Autodesk Inventor part; units mm, degrees
ref_plane "YZ Plane" through (0, 0, 0) normal (1, 0, 0) x (0, 1, 0)
ref_plane "XZ Plane" through (0, 0, 0) normal (0, 1, 0) x (-1, 0, 0)
ref_plane "XY Plane" through (0, 0, 0) normal (0, 0, 1) x (1, 0, 0)
sketch "Sketch2" plane through (0, 0, 0) normal (0, 1, 0) x (-1, 0, 0)
  line L0 (0, 0) -> (-30, 0)
  line L1 (-30, 0) -> (-30, -144)
  line L2 (-30, -144) -> (0, -144)
  line L3 (0, -144) -> (0, 0)
  line L4 (0, 0) -> (7, 0)
  line L5 (7, 0) -> (7, -5)
  arc A0 (7, -5) -> (0, -20.1987) centre (20, -20.1987) ccw
  line L6 (0, -144) -> (7, -144)
  line L7 (7, -144) -> (7, -139)
  arc A1 (0, -123.8013) -> (7, -139) centre (20, -123.8013) ccw
  line L8 (-30, 0) -> (-35, 0)
  line L9 (-35, 0) -> (-35, -52)
  line L10 (-35, -52) -> (-30, -52)
  line L11 (-30, -52) -> (-30, 0)
  line L12 (-30, -144) -> (-35, -144)
  line L13 (-35, -144) -> (-35, -92)
  line L14 (-35, -92) -> (-30, -92)
  line L15 (-30, -92) -> (-30, -144)
  line L16 (5, -32) -> (0, -32)
  line L17 (0, -52) -> (5, -52)
  line L18 (5, -52) -> (5, -32)
  line L19 (5, -92) -> (0, -92)
  line L20 (0, -112) -> (5, -112)
  line L21 (5, -112) -> (5, -92)
  dimension "d0" = 144
  dimension "d1" = 30
  dimension "d2" = 5
  dimension "d3" = 7
  dimension "d4" = 20
  dimension "d5" = 7
  dimension "d6" = 5
  dimension "d9" = 20
  dimension "d10" = 5
  dimension "d11" = 5
  dimension "d12" = 40
  dimension "d13" = 40
  dimension "d14" = 5
  dimension "d15" = 5
  dimension "d16" = 20
  dimension "d17" = 20
extrude "Cuerpo" add sketch "Sketch2" along normal blind 3
equation "\"d0\" = deslizador_largo"
equation "\"d1\" = deslizador_ancho"
equation "\"d2\" = deslizador_interruptor_largo"
equation "\"d3\" = deslizador_interruptor_ancho"
equation "\"d4\" = deslizador_interruptor_angulo"
equation "\"d5\" = d3"
equation "\"d6\" = d2"
equation "\"d9\" = d4"
equation "\"d10\" = deslizador_saliente"
equation "\"d11\" = d10"
equation "\"d12\" = movimiento_deslizador + deslizador_tope_largo"
equation "\"d13\" = d12"
equation "\"d14\" = d10"
equation "\"d15\" = d10"
equation "\"d16\" = deslizador_saliente_largo"
equation "\"d17\" = d16"
equation "\"d18\" = deslizador_alto"
equation "\"margen\" = 0.3"
equation "\"base_alto\" = 3"
equation "\"muros_grosor\" = 3"
equation "\"rail_alto\" = 1.5"
equation "\"rail_grosor\" = 5"
equation "\"hoja_stop_posicion\" = 5"
equation "\"hoja_stop_saliente\" = 5"
equation "\"hoja_stop_largo\" = 5"
equation "\"hoja_alto\" = 3"
equation "\"hoja_stop_biselado\" = 2"
equation "\"hoja_filo_biselado\" = 0.5"
equation "\"hoja_cola_biselado\" = 1"
equation "\"deslizador_soporte_alto\" = 4"
equation "\"deslizador_tope_alto\" = 5"
equation "\"deslizador_soporte_ancho\" = 5"
equation "\"deslizador_tope_largo\" = 10"
equation "\"deslizador_alto\" = 3"
equation "\"tirador_agarre_largo\" = 3"
equation "\"movimiento_deslizador\" = 30"
equation "\"deslizador_largo\" = 144"
equation "\"deslizador_ancho\" = 30"
equation "\"deslizador_saliente\" = 5"
equation "\"deslizador_interruptor_angulo\" = 20"
equation "\"deslizador_interruptor_largo\" = 5"
equation "\"deslizador_interruptor_ancho\" = 7"
equation "\"deslizador_saliente_largo\" = 20"
equation "\"traba_top_alto\" = 3"
equation "\"traba_top_largo\" = 5"
equation "\"traba_alto\" = 4"
equation "\"traba_ancho\" = 3"
equation "\"traba_largo\" = 39"
equation "\"traba_diametro\" = 5"
equation "\"traba_diametro_perforacion\" = 2"
equation "\"base_separacion_agujeros\" = 4"
equation "\"base_agujeros_separacion\" = 3.5"
equation "\"base_agujeros_diametro\" = 2"
properties part number "Deslizador"
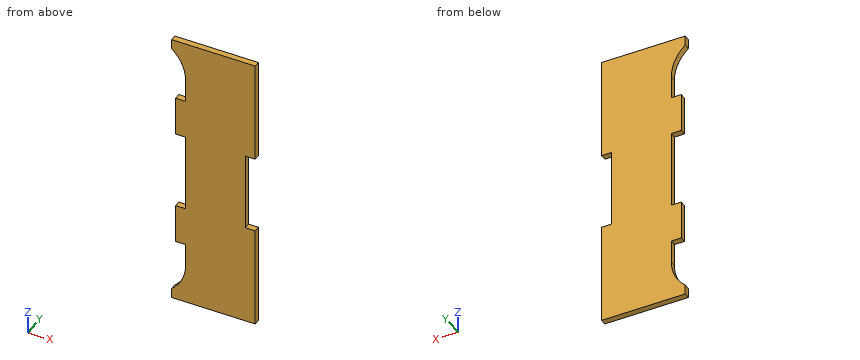
Geometry check sheet. Reference: the model listing, model coordinates, mm. Give positions to 0.01 mm unless a question says otherwise; leave off trailing zeros. Order: outer loops, then holes, each group sorted by start corner. A loop starts at its lowest first (then second) coordinate and runs counter-clockwise, first axis right, second up. Notation, with made-up numbers: (75, 43) - (115, 43) arc R22 ccw to (115, 49) - close; hole circle Ø5 at (-14, -38.5). An arc over 180 degrees is marked (long way). Answer as a JSON object with one key per item and string values.
(1) Material ranges on line 1 (Z direction, x = -2, y = 0.55); line 2 (X direction, y = 1.55, z = -74); line 3 (X direction, y = 2.75, z = -117), recorded low to high.
Report:
{"line 1": "-144 to -132.52, -112 to -92, -52 to -32, -11.48 to 0", "line 2": "0 to 30", "line 3": "0 to 35"}
(2) Cross-section at B-B (z = -34). Record the cut outline in (x, y), then the cut area to 3 significant figures.
Report:
{"outline": "(-5, 0) - (35, 0) - (35, 3) - (-5, 3) - close", "area": "120 mm^2"}
(3) Depth check by flat-ended pin: pin 1 Ø0.9 at (y, z) = (1, -98) entering from -X; pin 2 Ø8 at (x, z) = (14.5, -20.5) entering from -Y; pin 3 Ø1 at (x, z) = (-1.5, -121) entering from +Y; pin 4 Ø1.5 at (y, z) = (1.5, -80.5) entering from -X. Enter the tip coordinate at first touch or a pass-through.
Report:
{"pin 1": "x = -5", "pin 2": "y = 0", "pin 3": "through", "pin 4": "x = 0"}
(4) Cross-section at A-A (y = 2.05). Record the cut outline in (x, z), then the cut area to 3 significant figures.
Report:
{"outline": "(-7, -144) - (35, -144) - (35, -92) - (30, -92) - (30, -52) - (35, -52) - (35, 0) - (-7, 0) - (-7, -5) arc R20 cw to (0, -20.2) - (0, -32) - (-5, -32) - (-5, -52) - (0, -52) - (0, -92) - (-5, -92) - (-5, -112) - (0, -112) - (0, -123.8) arc R20 cw to (-7, -139) - close", "area": "5,180 mm^2"}
